```python
from build123d import *

# Parameters (mm, degrees)
F0_R     = 2.65
F1_DEPTH = 2.2
F0_W     = 1
F0_H     = 1.25
F0_W_2   = 1.25
F0_H_2   = 1
F2_DEPTH = 1
F3_R     = 0.5
F4_R     = 0.25
F5_R     = 1.52
F6_DEPTH = 15.26


with BuildPart() as f1:
    # F0 (on Front) → F1 (new body)
    with BuildSketch(Plane.XZ):
        Circle(F0_R)
        Polygon((0.5, -0.5), (0.5, -1.75), (-0.5, -1.75), (-0.5, -0.5), (-1.75, -0.5), (-1.75, 0.5), (-0.5, 0.5), (-0.5, 1.75), (0.5, 1.75), (0.5, 0.5), (1.75, 0.5), (1.75, -0.5), align=None, mode=Mode.SUBTRACT)
    extrude(amount=F1_DEPTH)

    # F0 (on Front) → F2 (join)
    with BuildSketch(Plane.XZ):
        with Locations((0, 1.125)):
            Rectangle(F0_W, F0_H)
        with Locations((1.125, 0)):
            Rectangle(F0_W_2, F0_H_2)
        with Locations((-1.125, 0)):
            Rectangle(F0_W_2, F0_H_2)
        Rectangle(F0_W, F0_H_2)
        with Locations((0, -1.125)):
            Rectangle(F0_W, F0_H)
    extrude(amount=F2_DEPTH)

    # F3
    f3_edges = [f1.edges().sort_by_distance(p)[0] for p in [
        (-2.65, -2.2, 0),
    ]]
    fillet(f3_edges, radius=F3_R)

    # F4
    f4_edges = [f1.edges().sort_by_distance(p)[0] for p in [
        (-2.65, 0, 0),
    ]]
    fillet(f4_edges, radius=F4_R)

    # F5 (on face) → F6 (join)
    with BuildSketch(Plane(origin=(0, 0, 0), x_dir=(-1, 0, 0), z_dir=(0, 1, 0))):
        Circle(F5_R)
    extrude(amount=F6_DEPTH)


solid = f1.part
```
Geometry: final body of the model. Coordinates: model frame, mm. A direction names the side the tool comes from. Give positions to 0.01 mm unless a question says otherwise; leave off trailing zeros. Write each loop counter-clockwise with the first axis right and the second up, starting at its lowest first coordinate (ties: lowest second). Pieces come first, ordered by that corner, then holes.
1. Section query B-B, the plane x = 0. Return loops of the section in (y, z), then the cut area to 3 significant figures.
2. Reachability of faces 1 (the flat face through (-1, -2, -0.5)), 2 (the cylindrical face through (-1.45, 7.52, 0.46)), 3 (the flat face through (0, 15.26, 0)) from +Z, -Z, +X, -X, +Y, -Y: full face, straight path, thin tool, end or side. Return the list, or none.
3. Section query C-C, the plane y = 8.75. Return loops of the section in (x, z), then the cut area to 3 significant figures.
4. Section query A-A, the plane z = 0. Return loops of the section in (x, y), then the cut area to 3 significant figures.
5. Draft query along Z for faces 4 (the flat face through (-1, -2.2, 1)), 5 (the flat face through (-1, -2, 0.5)), 6 (the cylindrical face through (2.45, -0.96, -1.01)). Return one class per face: released by +Z, released by -Z, zero draft, split by the parting line, or undercut.
6. Line query: probe 1 along Y at (x, z) = (0.25, 1); probe 2 along Y at (x, z) = (0.3, -2.05); probe 3 along X at (y, z) = (11.5, 0.05). Output: solid intervals per line, ascending.
7. Pin query (flat end, axial travel): P1, Ø0.5, axis at x = 0, y = -2, coming from the +Z side; P2, Ø0.6, axis at x = -1.5, y = -1.5, coming from the -Z side; P3, Ø0.6, axis at x = 1.5, y = -1.5, coming from the +Z side. Return the tip coordinate at first contact, or that it passes through.
Computed:
1. outline: (-2.2, -2.15) arc R0.5 ccw to (-1.7, -2.65) - (-0.25, -2.65) arc R0.25 ccw to (0, -2.4) - (0, -1.52) - (15.26, -1.52) - (15.26, 1.52) - (0, 1.52) - (0, 2.4) arc R0.25 ccw to (-0.25, 2.65) - (-1.7, 2.65) arc R0.5 ccw to (-2.2, 2.15) - (-2.2, 1.75) - (-1, 1.75) - (-1, -1.75) - (-2.2, -1.75) - close
1. area: 53.7 mm2
2. face 1: -Y
2. face 2: +Y
2. face 3: +Z, -Z, +X, -X, +Y
3. outline: circle Ø3.04 at (0, 0)
3. area: 7.26 mm2
4. outline: (-2.65, -1.7) arc R0.5 ccw to (-2.15, -2.2) - (-1.75, -2.2) - (-1.75, -1) - (1.75, -1) - (1.75, -2.2) - (2.15, -2.2) arc R0.5 ccw to (2.65, -1.7) - (2.65, -0.25) arc R0.25 ccw to (2.4, 0) - (1.52, 0) - (1.52, 15.26) - (-1.52, 15.26) - (-1.52, 0) - (-2.4, 0) arc R0.25 ccw to (-2.65, -0.25) - close
4. area: 53.7 mm2
5. face 4: zero draft
5. face 5: undercut
5. face 6: split by the parting line
6. probe 1: y = -1 to 15.26
6. probe 2: y = -2.2 to 0
6. probe 3: x = -1.52 to 1.52
7. P1: stops at z = 2.65
7. P2: stops at z = -2.36
7. P3: stops at z = 2.36
